```python
from build123d import *

# Parameters (mm, degrees)
SKETCH1_R           = 3.9
BOSS_EXTRUDE1_DEPTH = 270
BOSS_EXTRUDE2_DEPTH = 7.5


with BuildPart() as part:
    # Sketch1 → Boss-Extrude1 (new body)
    with BuildSketch(Plane(origin=(0, 0, 0), x_dir=(1, 0, 0), z_dir=(0, 1, 0))):
        with Locations(Location((0, 0, 0), (0, 0, 270))):
            Circle(SKETCH1_R)
    extrude(amount=BOSS_EXTRUDE1_DEPTH)

    # Sketch2 → Boss-Extrude2 (add)
    with BuildSketch(Plane(origin=(0, 270, 0), x_dir=(1, 0, 0), z_dir=(0, 1, 0))):
        Polygon((7.505553499, 0), (3.75277675, 6.5), (-3.75277675, 6.5), (-7.505553499, 0), (-3.75277675, -6.5), (3.75277675, -6.5), align=None)
    extrude(amount=BOSS_EXTRUDE2_DEPTH)

    # Sketch5 → Revolve2 (revolve)
    with BuildSketch(Plane(origin=(0, 0, 0), x_dir=(0.8660254037844384, 0, -0.5000000000000007), z_dir=(0.5000000000000006, 0, 0.8660254037844383))):
        with BuildLine():
            Line((0, 277.5), (6.5, 277.5))
            ThreePointArc((6.5, 277.5), (5.884153616, 280.261654617), (4.153311931, 282.5))
            Line((4.153311931, 282.5), (0, 282.5))
            Line((0, 282.5), (0, 277.5))
        make_face()
    revolve(axis=Axis((0, 282.5, 0), (0, -1, 0)))


solid = part.part
```
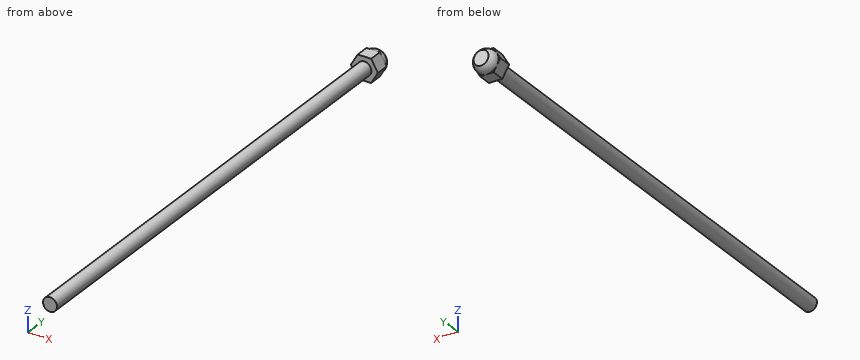
Verification items for the finished model (mm, model axes). Round coordinates to 2 decimals unless told otherwise and drop trailing zeros. Order: outer loops, then holes, each group sorted by start corner. A loop starts at its lowest first (then second) coordinate and runs counter-clockwise, first axis right, second up.
1) Material ranges on line 1 (X direction, y = 36, z = -1); line 2 (Y direction, x = -3.75, z = -6), recorded low to high.
Geometry says:
line 1: x = -3.77 to 3.77
line 2: y = 270 to 277.5
2) Depth check by flat-ended pin: pin 1 (1 mm diameter, centred on x = -5.5, y = 147, fed in from +Z); pin 2 (5 mm diameter, centred on y = 98.5, z = 0.5, fed in from -X); pin 3 (4 mm diameter, centred on x = -2.5, y = 171.5, fed in from -Z); pin 4 (1.5 mm diameter, centred on y = 134, z = 4, fed in from -X). Enter the tip coordinate at first touch or a pass-through.
Geometry says:
pin 1: passes through
pin 2: stops at x = -3.9
pin 3: stops at z = -3.87
pin 4: stops at x = -2.16
3) Cross-section at A-A, the plane y = 138. Record the cut outline in (x, z), plus the area to 3 significant figures.
Geometry says:
outline: circle Ø7.8 at (0, 0)
area: 47.8 mm2
